Here's how the part is built. I have some questions about the finished solid (model axes, mm). Face numbers are marked on the shaded views. Coordinates: 2 decimals unless noted, no trailing zeros. Write each loop counter-clockwise with the first axis right and the second up, starting at its lowest first coordinate (ties: lowest second). Pieces come first, ordered by that corner, then holes.
Item 1: I want a section at D-D (y = 9.5). Please give me the cut outline in (x, z).
Item 2: I want a section at C-C (y = 4). Please give me the cut outline in (x, z), and give its area (3 significant figures).
Item 3: Please list where these lines run through material, in increasing order: line 1 (X direction, y = 4.75, z = -0.5); line 2 (X direction, y = 9, z = 1); line 3 (X direction, y = 7.75, z = -5).
Item 4: If we mould it in two halves opening along Z, with no side actions, what happens to the marked faces 1 and 2? For each: pulls with the +Z half, pulls with the -Z half, needs draft (parallel to the pull), parting line crosses it, or undercut.
Item 5: I'm going to push flat-ended pins straight in: P1, Ø1, axis at y = 2.5, z = 6, coming from the -X side; P2, Ø10, axis at x = 11.5, z = -7, coming from the +Y side; P3, Ø4, axis at x = 0, z = 5, coming from the +Y side; P4, Ø5, axis at x = 5.5, y = 2, coming from the -Z side. Where does each tip first touch, or does it pass through?
Item 6: I want a section at A-A (x = 0). Count the separate pieces of the cut face and the enclosed holes in it, and give its area (3 significant figures).
from build123d import *

# Parameters (mm, degrees)
SKETCH_1_R      = 15
SKETCH_1_R_2    = 2.5
EXTRUDE_1_DEPTH = 10
FILLET_1_R      = 5


with BuildPart() as part:
    # 草图1 → 凸台-拉伸1 (new body)
    with BuildSketch(Plane(origin=(0, 0, 0), x_dir=(1, 0, 0), z_dir=(0, 1, 0))):
        with Locations(Location((0, 0, 0), (0, 0, 270))):
            Circle(SKETCH_1_R)
        with Locations(Location((0, 5, 0), (0, 0, 270))):
            Circle(SKETCH_1_R_2, mode=Mode.SUBTRACT)
        with Locations(Location((0, -5, 0), (0, 0, 270))):
            Circle(SKETCH_1_R_2, mode=Mode.SUBTRACT)
        with Locations(Location((5, 0, 0), (0, 0, 270))):
            Circle(SKETCH_1_R_2, mode=Mode.SUBTRACT)
        with Locations(Location((-5, 0, 0), (0, 0, 270))):
            Circle(SKETCH_1_R_2, mode=Mode.SUBTRACT)
    extrude(amount=EXTRUDE_1_DEPTH)

    # 圆角1
    fillet_1_edges = [part.edges().sort_by_distance(p)[0] for p in [
        (0, 0, -15),
        (0, 10, -15),
    ]]
    fillet(fillet_1_edges, radius=FILLET_1_R - 0.0001)  # a hair under: the kernel refuses the full size


solid = part.part
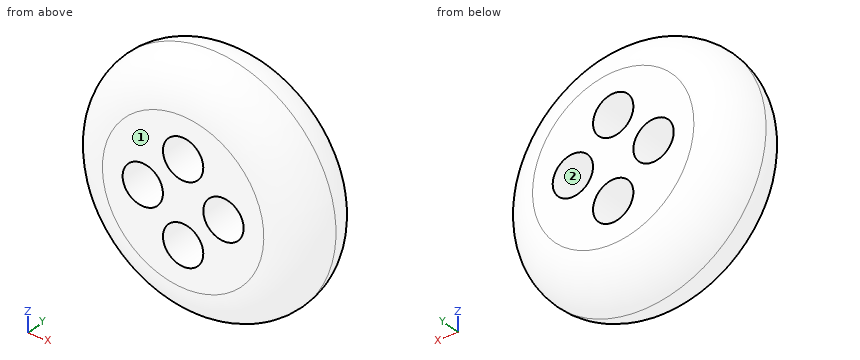
Answer:
1. outline: circle Ø24.36 at (0, 0); hole circle Ø5 at (-5, 0); hole circle Ø5 at (0, -5); hole circle Ø5 at (0, 5); hole circle Ø5 at (5, 0)
2. outline: circle Ø29.8 at (0, 0); hole circle Ø5 at (-5, 0); hole circle Ø5 at (0, -5); hole circle Ø5 at (0, 5); hole circle Ø5 at (5, 0)
2. area: 619 mm2
3. line 1: x = -14.99 to -7.45, -2.55 to 2.55, 7.45 to 14.99
3. line 2: x = -12.96 to -7.29, -2.71 to 2.71, 7.29 to 12.96
3. line 3: x = -13.26 to -2.5, 2.5 to 13.26
4. face 1: needs draft
4. face 2: undercut
5. P1: stops at x = -13.37
5. P2: stops at y = 10
5. P3: passes through
5. P4: stops at z = -14.37
6. separate pieces: 3
6. enclosed holes: 0
6. area: 179 mm2
